Work out the finished part from the listing and answer in its coordinate system (mm). Coordinates: 2 decimals unless noted, no trailing zeros. Loops run counter-clockwise (first coordinate to the right, second up) from the corner with the lowest first, then second, coordinate; pieces in that order, holes last. Notation, with made-up numbers: (11.25, -33.5) - (49.25, -33.5) arc R29 ccw to (49.25, -6.5) - close; hole circle Ø8 at (4, -15.75). An arc over 180 degrees is marked (long way). Write each question's results on one line, items separated by ' | '. Start each with the question number.
Item 1: Section D-D, the plane x = 7 is taken. Write down the section's boundary in (y, z) (3 decimals).
Item 2: Section B-B, the plane x = 13 is taken. Write down the section's boundary in (y, z) (3 decimals), plus the area to 3 significant figures.
Item 3: Section C-C, the plane y = -5.5 is taken. Write down the section's boundary in (x, z).
Item 4: This flat-tipped pin is pushed along its axis until it touches: pin 1 Ø1 at (x, y) = (16, -2) entering from +Z. Where does it stop, or does it pass through?
Item 5: Consider probe 1 along Y at (x, z) = (11.75, 0.35); probe 2 along Z at (x, y) = (21, -7.75); probe 3 along Y at (x, z) = (16.75, 0.6). Determine where each line is inside the solid, lowest interval first. Write a range as [from, to].
Item 6: Section A-A, the plane z = 0.85 is taken. Write down the section's boundary in (x, y).
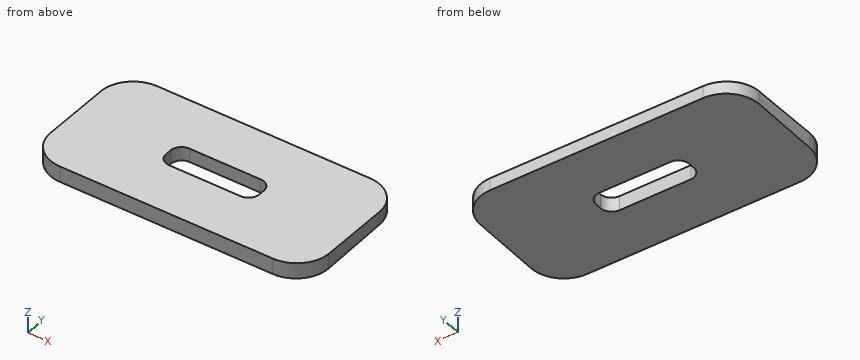
from build123d import *

# Parameters (mm, degrees)
PAD027_DEPTH    = 25.4
SKETCH051_W     = 2.6
SKETCH051_H     = 8.5
POCKET024_DEPTH = 2
FILLET022_R     = 3
FILLET023_R     = 1


with BuildPart() as part:
    # Sketch050 → Pad027 (new body)
    with BuildSketch(Plane.YZ):
        Polygon((0, 0), (-12.5, 0), (-12.5, 1.45), (0, 1.125), align=None)
    extrude(amount=PAD027_DEPTH)

    # Sketch051 (on Face1 of Pad027) → Pocket024 (cut)
    with BuildSketch(Plane.YX):
        with Locations((-6.25, 12.7)):
            Rectangle(SKETCH051_W, SKETCH051_H)
    extrude(amount=-POCKET024_DEPTH, mode=Mode.SUBTRACT)

    # Fillet022
    fillet022_edges = [part.edges().sort_by_distance(p)[0] for p in [
        (25.4, 0, 0.5625),
        (0, 0, 0.5625),
        (25.4, -12.5, 0.725),
        (0, -12.5, 0.725),
    ]]
    fillet(fillet022_edges, radius=FILLET022_R)

    # Fillet023
    fillet023_edges = [part.edges().sort_by_distance(p)[0] for p in [
        (16.95, -7.55, 0.66065),
        (8.45, -7.55, 0.66065),
        (8.45, -4.95, 0.62685),
        (16.95, -4.95, 0.62685),
    ]]
    fillet(fillet023_edges, radius=FILLET023_R)


solid = part.part
Answer key:
1) outline: (-12.5, 0) - (0, 0) - (0, 1.125) - (-12.5, 1.45) - close
2) outline: (-12.5, 0) - (-7.55, 0) - (-7.55, 1.321) - (-12.5, 1.45) - close; (-4.95, 0) - (0, 0) - (0, 1.125) - (-4.95, 1.254) - close | area: 12.7 mm^2
3) outline: (0, 0) - (8.56, 0) - (8.56, 1.27) - (0, 1.27) - close; (16.84, 0) - (25.4, 0) - (25.4, 1.27) - (16.84, 1.27) - close
4) pin 1: stops at z = 1.19
5) probe 1: y = [-12.5, -7.55], [-4.95, 0] | probe 2: z = [0, 1.33] | probe 3: y = [-12.5, -7.15], [-5.35, 0]
6) outline: (0, -9.5) arc R3 ccw to (3, -12.5) - (22.4, -12.5) arc R3 ccw to (25.4, -9.5) - (25.4, -3) arc R3 ccw to (22.4, 0) - (3, 0) arc R3 ccw to (0, -3) - close; hole (8.45, -6.55) arc R1 ccw to (9.45, -7.55) - (15.95, -7.55) arc R1 ccw to (16.95, -6.55) - (16.95, -5.95) arc R1 ccw to (15.95, -4.95) - (9.45, -4.95) arc R1 ccw to (8.45, -5.95) - close
